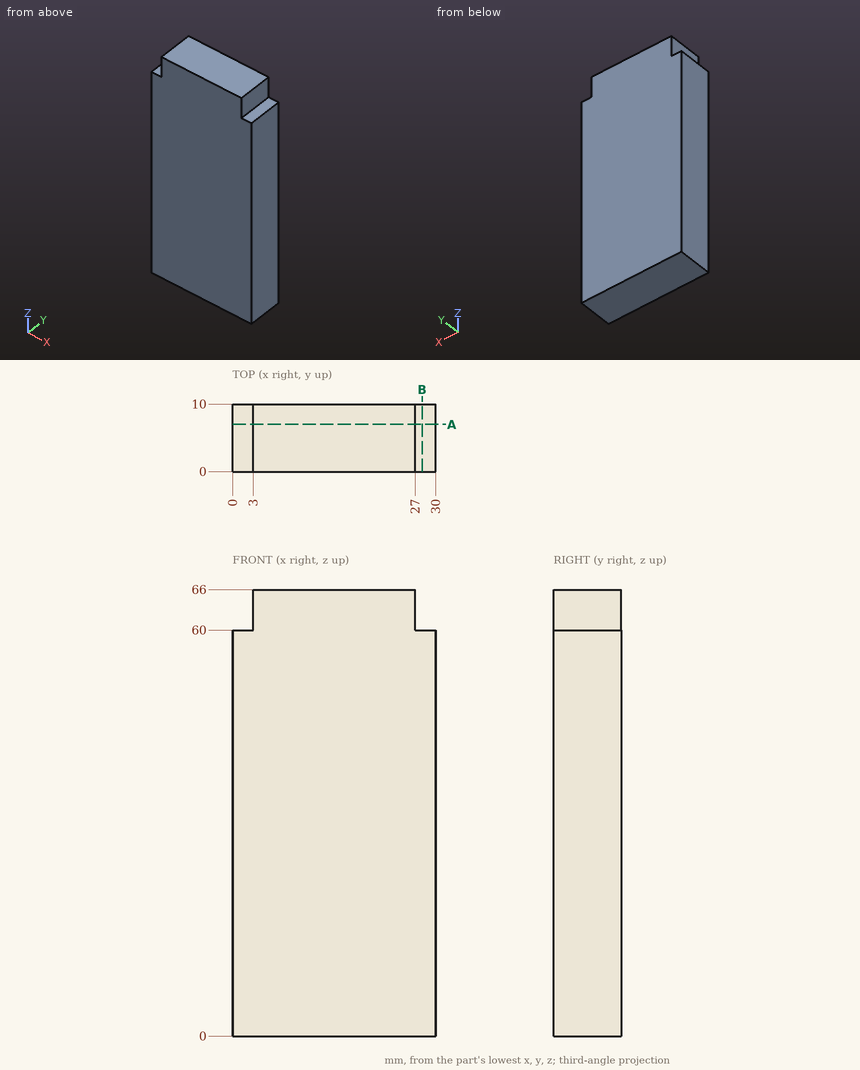
Could you check a few things on this drawing? It's one solid part, dimensions in mm from its lowest x, y, z. Coordinates: 2 decimals unless noted, no trailing zeros. Loops run counter-clockwise (first coordinate to the right, second up) from the corner with the lowest first, then second, coordinate; pieces in that order, holes last. Notation, with made-up numbers: (50, 87.25) - (56, 87.25) arc R27 cw to (56, 110.25) - close; hole circle Ø1 at (81, 51.5). An arc over 180 degrees is marked (long way). Return JSON: item names as keys, results as strings. Group by question number.
Item 1: I need wall thicknesses on line 1 (Z direction, x = 28.5, y = 4). Which ranges of the line are inside material? Lowest first, please. Write a range as from..to.
Item 2: Will these pins go through, and if not, where does the flat tip stop? P1, Ø3, axis at y = 5, z = 64, coming from the +X side; P2, Ø3, axis at y = 2.5, z = 64, coming from the -X side; P3, Ø1.5, axis at x = 28.5, y = 6.5, coming from the +Z side.
Item 3: If we section it at B-B on x = 28: Write out the boundary of the cut face in (y, z).
Item 4: If we section it at A-A on y = 7: Write out the boundary of the cut face in (x, z), and give its area (3 significant figures).
Calculated:
{
 "1": {"line 1": "z = 0..60"},
 "2": {"P1": "stops at x = 27", "P2": "stops at x = 3", "P3": "stops at z = 60"},
 "3": {"outline": "(0, 0) - (10, 0) - (10, 60) - (0, 60) - close"},
 "4": {"outline": "(0, 0) - (30, 0) - (30, 60) - (27, 60) - (27, 66) - (3, 66) - (3, 60) - (0, 60) - close", "area": "1,940 mm^2"}
}
